from build123d import *

# Parameters (mm, degrees)
SKETCH1_W            = 29.9
SKETCH1_H            = 10.3
SKETCH1_R            = 2.4
BOSS_EXTRUDE1_DEPTH  = 30
BOSS_EXTRUDE3_START  = -2
SKETCH4_W            = 29.9
SKETCH4_H            = 10.3
BOSS_EXTRUDE3_DEPTH  = 28
SKETCH2_W            = 20.9
SKETCH2_H            = 25
CUT_EXTRUDE1_DEPTH   = 11.3
SKETCH3_W            = 0.8
SKETCH3_H            = 3
CUT_EXTRUDE2_DEPTH   = 31
M3_CLEARANCE_HOLE1_D = 3.6
SKETCH7_W            = 1.2265006
SKETCH7_H            = 3
SKETCH7_W_2          = 1.1265006
CUT_EXTRUDE3_DEPTH   = 2
CUT_EXTRUDE4_DEPTH   = 2
CHAMFER1_SIZE        = 0.6


with BuildPart() as part:
    # Sketch1 → Boss-Extrude1 (new body)
    with BuildSketch(Plane(origin=(0, 0, 0), x_dir=(1, 0, 0), z_dir=(0, 1, 0))):
        with Locations((-5.3, 0)):
            Rectangle(SKETCH1_W, SKETCH1_H)
        Circle(SKETCH1_R, mode=Mode.SUBTRACT)
        with Locations((-14.25, 0)):
            Circle(SKETCH1_R, mode=Mode.SUBTRACT)
    extrude(amount=BOSS_EXTRUDE1_DEPTH)

    # Sketch4 → Boss-Extrude3 (add)
    with BuildSketch(Plane.XZ.offset(BOSS_EXTRUDE3_START)):
        with Locations((-5.3, 0)):
            Rectangle(SKETCH4_W, SKETCH4_H)
    extrude(amount=-BOSS_EXTRUDE3_DEPTH)

    # Sketch2 → Cut-Extrude1 (cut, through all)
    with BuildSketch(Plane.XY.offset(5.15)):
        with Locations((-9.8, 17.5)):
            Rectangle(SKETCH2_W, SKETCH2_H)
    extrude(amount=-CUT_EXTRUDE1_DEPTH, mode=Mode.SUBTRACT)

    # Sketch3 → Cut-Extrude2 (cut, through all)
    with BuildSketch(Plane.XZ):
        with Locations((-11.55, 0)):
            Rectangle(SKETCH3_W, SKETCH3_H)
        with Locations((-2.6, 0)):
            Rectangle(SKETCH3_W, SKETCH3_H)
    extrude(amount=-CUT_EXTRUDE2_DEPTH, mode=Mode.SUBTRACT)

    # M3 Clearance Hole1 (through all)
    with Locations(Plane.XY.offset(5.15)):
        with Locations((4.65, 12), (4.65, 27)):
            Hole(M3_CLEARANCE_HOLE1_D / 2)

    # Sketch7 → Cut-Extrude3 (cut)
    with BuildSketch(Plane.XZ):
        with Locations((-11.7632503, 0)):
            Rectangle(SKETCH7_W, SKETCH7_H)
        with Locations((-2.4367497, 0)):
            Rectangle(SKETCH7_W_2, SKETCH7_H)
    extrude(amount=-CUT_EXTRUDE3_DEPTH, mode=Mode.SUBTRACT)

    # Sketch8 → Cut-Extrude4 (cut)
    with BuildSketch(Plane.XZ):
        Polygon((-15.635640646, 2.4), (-17.021281292, 0), (-15.635640646, -2.4), (-12.864359354, -2.4), (-11.478718708, 0), (-12.864359354, 2.4), align=None)
        Polygon((1.385640646, 2.4), (-1.385640646, 2.4), (-2.771281292, 0), (-1.385640646, -2.4), (1.385640646, -2.4), (2.771281292, 0), align=None)
    extrude(amount=-CUT_EXTRUDE4_DEPTH, mode=Mode.SUBTRACT)

    # Chamfer1
    chamfer1_edges = [part.edges().sort_by_distance(p)[0] for p in [
        (-11.747372056, 0, -1.5),
        (-2.452627944, 0, 1.5),
        (-12.604551733, 0, 1.95),
        (-14.25, 0, 2.4),
        (-16.328460969, 0, 1.2),
        (-16.328460969, 0, -1.2),
        (-14.25, 0, -2.4),
        (-12.604551733, 0, -1.95),
        (-1.645448267, 0, 1.95),
        (0, 0, 2.4),
        (2.078460969, 0, 1.2),
        (2.078460969, 0, -1.2),
        (0, 0, -2.4),
        (-1.645448267, 0, -1.95),
        (-5.3, 0, -5.15),
        (9.65, 0, 0),
        (-5.3, 0, 5.15),
        (-20.25, 0, 0),
        (-11.15, 0, 0),
        (-11.747372056, 0, 1.5),
        (-3, 0, 0),
        (-2.452627944, 0, -1.5),
    ]]
    chamfer(chamfer1_edges, length=CHAMFER1_SIZE)


solid = part.part
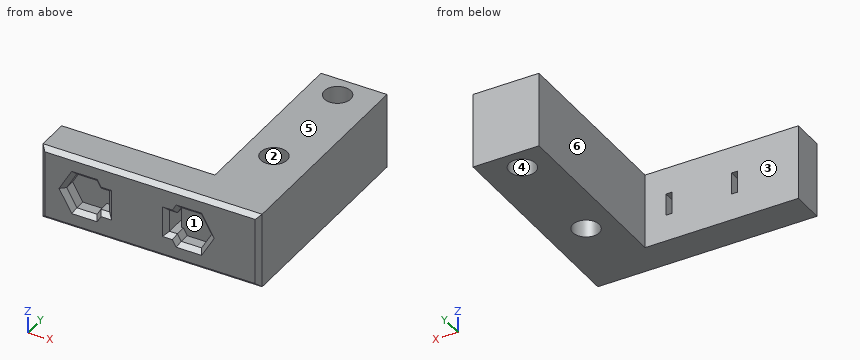
Geometry check sheet. Reference: the model listing, model coordinates, mm. Face numbers are marked on the shaded views. A direction names the side the tool comes from. Round coordinates to 2 decimals unless told otherwise and drop trailing zeros. Order: outer loops, then holes, each group sorted by start corner. A loop starts at its lowest first (then second) coordinate and runs counter-clockwise, first axis right, second up. Notation, with made-up numbers: M 63.5,10 L 114.5,10 A25 cw 114.5,32 Z; hole C -2.75,-16.75 d11. An arc over 180 degrees is marked long. Answer in a Markdown table with one row per item. Add a question column.
Item 1: Sectioned sample at C-C, the plane x = -0.25. Enter the section's corners in (y, z), plus the area to 3 significant figures.
Item 2: Material ranges on L1, parallel to Y at x = 4.65, z = -1.75; L2, parallel to Y at x = -4.25, z = 2.75; L3, parallel to Y at x = -14, z = 2.25, recorded low to high. Write a range as [from, to].
Item 3: Draft check along X on the marked faces 4, 5 and 6. Enter one of: released by +X, released by -X, zero draft, split by the parting line, or undercut.
Item 4: Sectioned sample at D-D, the plane y = 19.5. Enter the section's corners in (x, z).
Item 5: Set-up check for the marked faces 1, 2 and 3: record each of +Z, -Z, +X, -X, +Y, -Y from which the full face is reachable in a straight line by a thin tool's end or side.
Item 6: Depth check by flat-ended pin: pin 1 Ø3 at (y, z) = (23.5, 1) entering from -X; pin 2 Ø2.5 at (x, z) = (-15.5, 0) entering from -Y. Enter the tip coordinate at first touch or a pass-through.
Item 7: Sectioned sample at B-B, the plane x = 4.65. Enter the section's corners in (y, z), plus the area to 3 significant figures.
Item 8: Sectioned sample at A-A, the plane y = 27. Enter the section's corners in (x, z).
Filled in:
| question | item | result |
|---|---|---|
| 1 | outline | M 0,-4.55 L 0.6,-5.15 L 5,-5.15 L 5,5.15 L 0.6,5.15 L 0,4.55 L 0,3 L 0.6,2.4 L 2,2.4 L 2,-2.4 L 0.6,-2.4 L 0,-3 Z |
| 1 | area | 41.2 mm² |
| 2 | L1 | y = [0, 10.2], [13.8, 25.2], [28.8, 30] |
| 2 | L2 | y = [0, 5] |
| 2 | L3 | y = [2, 5] |
| 3 | face 4 | undercut |
| 3 | face 5 | zero draft |
| 3 | face 6 | released by -X |
| 4 | outline | M 0.65,-5.15 L 9.65,-5.15 L 9.65,5.15 L 0.65,5.15 Z |
| 5 | face 1 | -Y |
| 5 | face 2 | +Z, -Z |
| 5 | face 3 | +Z, -Z, -X, +Y |
| 6 | pin 1 | stops at x = 0.65 |
| 6 | pin 2 | stops at y = 2 |
| 7 | outline | M 0,-4.55 L 0.6,-5.15 L 10.2,-5.15 L 10.2,5.15 L 0.6,5.15 L 0,4.55 Z; M 13.8,-5.15 L 25.2,-5.15 L 25.2,5.15 L 13.8,5.15 Z; M 28.8,-5.15 L 30,-5.15 L 30,5.15 L 28.8,5.15 Z |
| 7 | area | 234 mm² |
| 8 | outline | M 0.65,-5.15 L 2.85,-5.15 L 2.85,5.15 L 0.65,5.15 Z; M 6.45,-5.15 L 9.65,-5.15 L 9.65,5.15 L 6.45,5.15 Z |
